Part model, mm, in its own coordinate system. A direction names the side the tool comes from. Round coordinates to 2 decimals unless told otherwise and drop trailing zeros. Loops run counter-clockwise (first coordinate to the right, second up) from the corner with the lowest first, then second, coordinate; pieces in that order, holes last.
from build123d import *

# Parameters (mm, degrees)
SKETCH1_R             = 85
BOSS_EXTRUDE1_DEPTH   = 4
SKETCH2_R             = 15
CUT_EXTRUDE1_DEPTH    = 121.274685616
SKETCH3_R             = 1.987487824
CUT_EXTRUDE2_DEPTH    = 2.677604
CIRPATTERN1_START     = 1.322395983
CIRPATTERN1_OUTLINE_R = 1.987487824
CIRPATTERN1_DEPTH     = 2.677604017


# Read off the part's stored shape, not the designer's step: CirPattern1
with BuildPart() as part:
    # Sketch1 → Boss-Extrude1 (new body)
    with BuildSketch(Plane(origin=(0, 0, 0), x_dir=(1, 0, 0), z_dir=(0, 1, 0))):
        with Locations(Location((0, 0, 0), (0, 0, 270))):
            Circle(SKETCH1_R)
    extrude(amount=BOSS_EXTRUDE1_DEPTH)

    # Sketch2 → Cut-Extrude1 (cut, through all)
    with BuildSketch(Plane(origin=(0, 0, 0), x_dir=(1, 0, 0), z_dir=(0, 1, 0))):
        with Locations(Location((0, 0, 0), (0, 0, 270))):
            Circle(SKETCH2_R)
    extrude(amount=CUT_EXTRUDE1_DEPTH, mode=Mode.SUBTRACT)

    # Sketch3 → Cut-Extrude2 (cut)
    with BuildSketch(Plane(origin=(0, 4, 0), x_dir=(1, 0, 0), z_dir=(0, 1, 0))):
        with Locations(Location((-26.539929768, 0, 0), (0, 0, 270))):
            Circle(SKETCH3_R)
    extrude(amount=-CUT_EXTRUDE2_DEPTH, mode=Mode.SUBTRACT)

    # CirPattern1 outline → CirPattern1 (cut)
    with BuildSketch(Plane(origin=(0, 0, 0), x_dir=(1, 0, 0), z_dir=(0, 1, 0)).offset(CIRPATTERN1_START)):
        with Locations((-13.269964884, -22.984253394)):
            Circle(CIRPATTERN1_OUTLINE_R)
        with Locations((13.269964884, -22.984253394)):
            Circle(CIRPATTERN1_OUTLINE_R)
        with Locations((26.539929768, 0)):
            Circle(CIRPATTERN1_OUTLINE_R)
        with Locations((13.269964884, 22.984253394)):
            Circle(CIRPATTERN1_OUTLINE_R)
        with Locations((-13.269964884, 22.984253394)):
            Circle(CIRPATTERN1_OUTLINE_R)
    extrude(amount=CIRPATTERN1_DEPTH, mode=Mode.SUBTRACT)


solid = part.part
1) Mould opens along Z. For faces 3 (the face through (-27, 1.322, 0)), 4 (the face through (-51.721, 1.972, -67.453)), 5 (the face through (-18, 0, -1)), 6 (the face through (-12.2, 2.64, -24.66)) say: released by +Z, released by -Z, zero draft, split by the parting line, or undercut.
Values:
face 3: undercut
face 4: split by the parting line
face 5: zero draft
face 6: undercut
2) Drop flat-ended pins along their axis: pin 1 Ø3 at (x, z) = (26.5, 1) entering from +Y; pin 2 Ø2.5 at (x, z) = (26.54, 0) entering from +Y. Give the stop position or say it passes through.
Values:
pin 1: stops at y = 4
pin 2: stops at y = 1.32
3) Slice it at D-D, the plane z = 36. Give the cut face in (x, y), then the cut area to 3 significant figures.
Values:
outline: (-77, 0) - (77, 0) - (77, 4) - (-77, 4) - close
area: 616 mm2
4) Wall check: line 1 along X through (y, z) = (2.75, 0); line 2 along Z through (x, y) = (-5, 3.8); line 3 along Z through (x, y) = (-28, 2.9). Give the ranges that are in metal, low to high.
Values:
line 1: x = -85 to -28.53, -24.55 to -15, 15 to 24.55, 28.53 to 85
line 2: z = -84.85 to -14.14, 14.14 to 84.85
line 3: z = -80.26 to -1.35, 1.35 to 80.26
5) Slice it at B-B, the plane x = 0. Give the cut face in (y, z), then the cut area to 3 significant figures.
Values:
outline: (0, -85) - (4, -85) - (4, -15) - (0, -15) - close; (0, 15) - (4, 15) - (4, 85) - (0, 85) - close
area: 560 mm2
6) Tool access for faces 1 (the face through (-24.57, 2.68, -0.26)), 2 (the face through (0.66, 1.972, -14.985)): list every direction of +Z, -Z, +X, -X, +Y, -Y with a clear straight run to the whole face (end or side of a thin tool).
Values:
face 1: +Y
face 2: +Y, -Y
7) Slice it at C-C, the plane y = 0.7. Give the cut face in (x, z).
Values:
outline: circle Ø170 at (0, 0); hole circle Ø30 at (0, 0)
8) Slice it at A-A, the plane z = 0. Give the cut face in (x, y).
Values:
outline: (-85, 0) - (-15, 0) - (-15, 4) - (-24.55, 4) - (-24.55, 1.32) - (-28.53, 1.32) - (-28.53, 4) - (-85, 4) - close; (15, 0) - (85, 0) - (85, 4) - (28.53, 4) - (28.53, 1.32) - (24.55, 1.32) - (24.55, 4) - (15, 4) - close
